Geometry: final body of the model. Coordinates: model frame, mm. A direction names the side the tool comes from. Give positions to 0.01 mm unless a question says otherwise; leave off trailing zeros. Write each loop counter-clockwise with the first axis right and the second up, starting at its lowest first coordinate (ties: lowest second). Pieces come first, ordered by that corner, then holes.
Q1. Section A-A (z = 18.5). Return the cut outline in (x, y), plus the area to 3 significant figures.
Q2. Section B-B (x = -6). Return the cut outline in (y, z).
Q3. Section C-C (y = -4.95). State how many separate pieces and enclosed holes the cut face has, plus the area to 3 significant figures.
Q4. Mould query, pull axis X, two halves, no side actions, for faces 1 (the flat face through (42.7, -3, -23)), 2 (the flat face through (23, -3, 42.7)), 3 (the cylindrical face through (-30.22, -3.04, 35.31)). Classes: +X half, -X half, draft (parallel to the pull), parting line (faces both ways), or undercut.
Q5. Line query: line 1 (Z direction, x = -34, y = -5.7); line 2 (X direction, y = -4.7, z = 33); line 3 (Z direction, x = -35, y = -4.7). Output: solid intervals per line, ascending.
Q6. Pin query (flat end, axial travel): pin 1 Ø3 at (x, y) = (-52.5, -3.5) entering from +Z; pin 2 Ø3.5 at (x, z) = (-30.19, 32.31) entering from -Y; pin 3 Ø1.8 at (y, z) = (-3.5, -32.5) entering from +X; pin 4 Ø2.5 at (x, z) = (-32.31, -30.19) entering from -Y. Return the tip coordinate at first contact, or that it passes through.
Q7. Reachability of faces 4 (the flat face through (46.5, -3.04, 13.89)), 5 (the flat face through (-54, -3, 0)), 6 (the flat face through (0, -3, 54)) from +Z, -Z, +X, -X, +Y, -Y: full face, straight path, thin tool, end or side. Return the list, or none.
from build123d import *

# Parameters (mm, degrees)
F0_R            = 60
F2_DEPTH        = 6
F4_D            = 3
F4_COPIES_COUNT = 8
F6_DEPTH        = 25
F6_COPIES_COUNT = 8


# Not quite as in the source:
# - a pattern or mirror of a feature is missing from the dataset's text; its kind, count and spacing are read off the source's solid


with BuildPart() as f2:
    # F0 (on Front) → F2 (new body)
    with BuildSketch(Plane.XZ):
        Circle(F0_R)
    extrude(amount=F2_DEPTH)

    # F4 (through all)
    with Locations(Plane.XZ.offset(6)):
        with Locations((1.5, 44.1936596632)):
            f4 = Hole(F4_D / 2)

    # F4_copies: F4 ×8 about axis
    f4_copies_axis = Axis((0, 0, 0), (0, 1, 0))
    for i in range(1, F4_COPIES_COUNT):
        add(f4.rotate(f4_copies_axis, i * 360 / F4_COPIES_COUNT), mode=Mode.SUBTRACT)

    # F5 (on face) → F6 (cut)
    with BuildSketch(Plane.XZ.offset(6)):
        with BuildLine():
            Line((4.5, 44.1936596632), (4.5, 42.7004098892))
            Line((4.5, 42.7004098892), (42.1506227154, 42.7004098892))
            ThreePointArc((42.1506227154, 42.7004098892), (22.7813016161, 55.5068671128), (0, 60))
            Line((0, 60), (0, 47.1936596632))
            Line((0, 47.1936596632), (1.5, 47.1936596632))
            ThreePointArc((1.5, 47.1936596632), (3.6213203436, 46.3149800068), (4.5, 44.1936596632))
        make_face()
        with BuildLine():
            ThreePointArc((0, 60), (22.7813016161, 55.5068671128), (42.1506227154, 42.7004098892))
            Line((42.1506227154, 42.7004098892), (58.9860603213, 42.7004098892))
            Line((58.9860603213, 42.7004098892), (58.9860603213, 64.2154142261))
            Line((58.9860603213, 64.2154142261), (0, 64.2154142261))
            Line((0, 64.2154142261), (0, 60))
        make_face()
    f6 = extrude(amount=-F6_DEPTH, mode=Mode.SUBTRACT)

    # F6_copies: F6 ×8 about axis
    f6_copies_axis = Axis((0, 0, 0), (0, 1, 0))
    for i in range(1, F6_COPIES_COUNT):
        add(f6.rotate(f6_copies_axis, i * 360 / F6_COPIES_COUNT), mode=Mode.SUBTRACT)


solid = f2.part
Computed:
1. outline: (-42.7, -6) - (41.89, -6) - (41.89, 0) - (-42.7, 0) - close
1. area: 508 mm2
2. outline: (-6, -42.7) - (0, -42.7) - (0, 54.39) - (-6, 54.39) - close
3. separate pieces: 1
3. enclosed holes: 8
3. area: 7,380 mm2
4. face 1: +X half
4. face 2: draft
4. face 3: undercut
5. line 1: z = -42.7 to -34, -32.74 to -27.64, -26.39 to 34
5. line 2: x = -42.7 to -31.52, -28.86 to 33.74
5. line 3: z = -42.7 to -35, -31.52 to -28.86, -25.39 to 35
6. pin 1: stops at z = 0
6. pin 2: stops at y = -6
6. pin 3: stops at x = 42.7
6. pin 4: passes through
7. face 4: +X, +Y, -Y
7. face 5: +Z, -X, +Y, -Y
7. face 6: +Z, +X, +Y, -Y
